Part model, mm, in its own coordinate system. A direction names the side the tool comes from. Round coordinates to 2 decimals unless told otherwise and drop trailing zeros. Loops run counter-clockwise (first coordinate to the right, second up) from the corner with the lowest first, then second, coordinate; pieces in that order, holes last.
(1) Cut at D-D on y = 34. List the corners of the cut face in (x, z), then the cut area to 3 significant figures.
(2) Tool access for faces 1 (the face through (33, -24, 6)), 2 (the face through (-24, -23, 6)), 3 (the face through (-15, 24, 6)), 4 (the face through (-24, 25, 6)): list every direction of +Z, -Z, +X, -X, +Y, -Y with a clear straight run to the whole face (end or side of a thin tool).
(3) Cut at C-C on x = 13.5. List the corners of the cut face in (y, z).
(4) Flat gauge pins, fed straight in: pin 1 (0.6 mm diameter, centred on x = 23.5, z = 6, fed in from -Y); pin 2 (0.6 mm diameter, centred on x = 21.5, z = 6.5, fed in from +Y); pin 3 (0.6 mm diameter, centred on y = -23.5, z = 6, fed in from +X). Where does each tip first touch, or does it go through?
(5) Cut at A-A on x = 25. List the corners of the cut face in (y, z), then the cut area to 3 significant figures.
(6) Mould opens along Y. For faces 5 (the face through (24, -23, 6)), 6 (the face through (24, 23, 6)), 7 (the face through (24, 25, 6)), 8 (the face through (-33.859, -0.504, 1.203)) say: +Y half, -Y half, draft (parallel to the pull), parting line (faces both ways), or undercut.
(7) Probe probe 1 along Y at (x, z) = (-25, 3.85); probe 2 along Y at (x, z) = (-13.5, 3.65); probe 3 along Y at (x, z) = (-25, 2.25). List the from-to ranges inside material, lowest first.
(8) Cut at B-B on y = 0. List the corners of the cut face in (x, z).
Solid Edge part; units mm, degrees
sketch "Sketch1" plane through (0, 0, 0) normal (0, 0, 1) x (1, 0, 0)
  line L0 (-35, -40) -> (35, -40)
  line L1 (35, -40) -> (35, 40)
  line L2 (35, 40) -> (-35, 40)
  line L3 (-35, 40) -> (-35, -40)
  dimension "D1" = 35
  dimension "D2" = 35
extrude "Protrusion1" add sketch "Sketch1" along normal blind 5
sketch "Sketch2" plane through (0, 0, 5) normal (0, 0, 1) x (1, 0, 0)
  circle A0 centre (-25, 34) radius 1.6
  dimension "D1" = 25
extrude "Cutout1" cut sketch "Sketch2" against normal through all
mirror "Mirror1" about plane through (0, 0, 0) normal (1, 0, 0) of "Cutout1"
mirror "Mirror2" about plane through (0, 0, 0) normal (0, -1, 0) of "Cutout1", "Mirror1"
sketch "Sketch3" plane through (0, 0, 5) normal (0, 0, 1) x (1, 0, 0)
  circle A0 centre (-13.5, 0) radius 1.5
extrude "Cutout2" cut sketch "Sketch3" against normal through all
mirror "Mirror3" about plane through (0, 0, 0) normal (1, 0, 0) of "Cutout2"
sketch "Sketch4" plane through (0, 0, 5) normal (0, 0, 1) x (1, 0, 0)
  line L0 (-33, 23) -> (-15, 23)
  line L1 (-15, 23) -> (-15, 25)
  line L2 (-15, 25) -> (-33, 25)
  line L3 (-33, 25) -> (-33, 23)
  dimension "D1" = 15
  dimension "D2" = 15
extrude "Extrusionsausprägung_2" add sketch "Sketch4" along normal blind 2
mirror "Mirror4" about plane through (0, 0, 0) normal (0, -1, 0) of "Extrusionsausprägung_2"
mirror "Mirror5" about plane through (0, 0, 0) normal (1, 0, 0) of "Mirror4", "Extrusionsausprägung_2"
fillet "Verrundung_1" radius 4 4 edges at (0, 40, 0) (35, 0, 0) (-35, 0, 0) (0, -40, 0)
fillet "Verrundung_2" radius 4 8 edges at (33.8284, 38.8284, 1.1716) (35, 40, 4.5) (33.8284, -38.8284, 1.1716) (35, -40, 4.5) (-33.8284, -38.8284, 1.1716) (-35, -40, 4.5) (-33.8284, 38.8284, 1.1716) (-35, 40, 4.5)
properties material "Nylon, allgemein"
Final values:
1. outline: (-35, 4) arc R4 ccw to (-31, 0) - (-26.6, 0) - (-26.6, 5) - (-35, 5) - close; (-23.4, 0) - (23.4, 0) - (23.4, 5) - (-23.4, 5) - close; (26.6, 0) - (31, 0) arc R4 ccw to (35, 4) - (35, 5) - (26.6, 5) - close
1. area: 311 mm2
2. face 1: +Z, +X, +Y, -Y
2. face 2: +Z, +X, -X
2. face 3: +Z, +Y, -Y
2. face 4: +Z, +X, -X, +Y
3. outline: (-40, 4) arc R4 ccw to (-36, 0) - (-1.5, 0) - (-1.5, 5) - (-40, 5) - close; (1.5, 0) - (36, 0) arc R4 ccw to (40, 4) - (40, 5) - (1.5, 5) - close
4. pin 1: stops at y = -25
4. pin 2: stops at y = 25
4. pin 3: stops at x = 33
5. outline: (-40, 4) arc R4 ccw to (-36, 0) - (-35.6, 0) - (-35.6, 5) - (-40, 5) - close; (-32.4, 0) - (32.4, 0) - (32.4, 5) - (25, 5) - (25, 7) - (23, 7) - (23, 5) - (-23, 5) - (-23, 7) - (-25, 7) - (-25, 5) - (-32.4, 5) - close; (35.6, 0) - (36, 0) arc R4 ccw to (40, 4) - (40, 5) - (35.6, 5) - close
5. area: 369 mm2
6. face 5: undercut
6. face 6: undercut
6. face 7: +Y half
6. face 8: draft
7. probe 1: y = -40 to -35.6, -32.4 to 32.4, 35.6 to 40
7. probe 2: y = -39.98 to -1.5, 1.5 to 39.98
7. probe 3: y = -39.6 to -35.6, -32.4 to 32.4, 35.6 to 39.6
8. outline: (-35, 4) arc R4 ccw to (-31, 0) - (-15, 0) - (-15, 5) - (-35, 5) - close; (-12, 0) - (12, 0) - (12, 5) - (-12, 5) - close; (15, 0) - (31, 0) arc R4 ccw to (35, 4) - (35, 5) - (15, 5) - close
